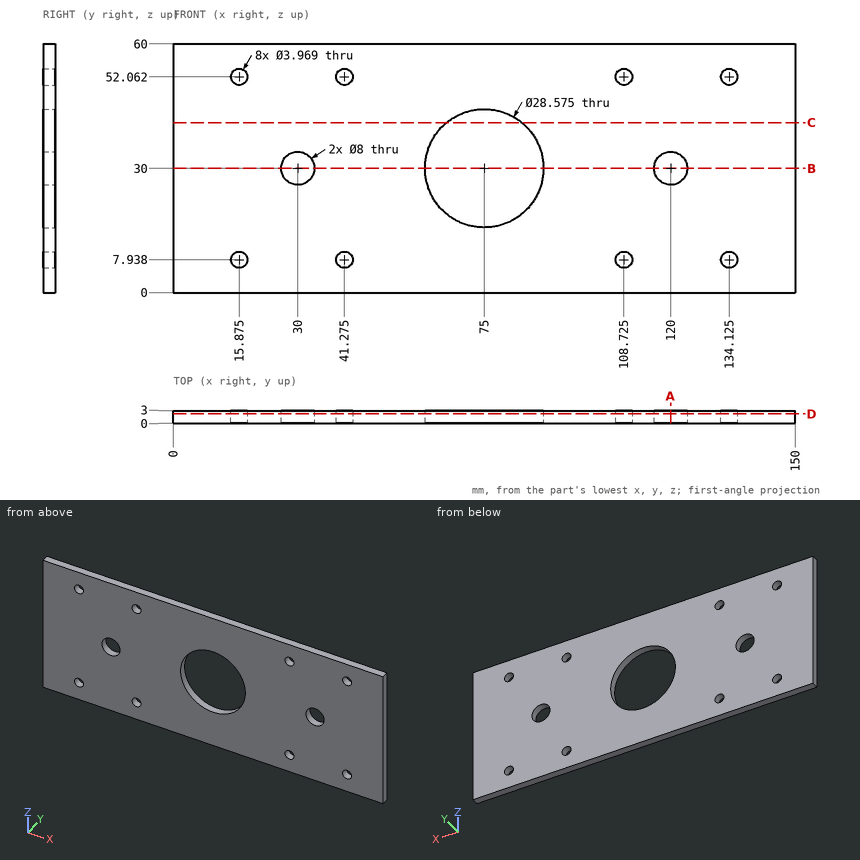
Print and shaded views of the part. All mm, measured from the part's lowest x, y and z. Round coordinates to 2 decimals unless told otherwise and drop trailing zeros. Order: outer loops, then holes, each group sorted by start corner. A loop starts at its lowest first (then second) coordinate and runs counter-clockwise, first axis right, second up.
Q1. Slice it at B-B (z = 30). Write the cut outline in (x, y).
Q2. Slice it at A-A (x = 120). Write the cut outline in (y, z), and give its area (3 significant figures).
Q3. Drop a flat-ended pin along its axis: pin 1 (5 mm diameter, centred on x = 134.12, z = 7.94, fed in from -Y). Give the stop position or say it passes through.
Q4. Wall check: L1, parallel to X at y = 1.9, z = 52; L2, parallel to X at y = 1.45, z = 30; L3, parallel to Z at x = 30, y = 0.75. Give the ranges that are in metal, low to high.
Q5. Slice it at D-D (y = 2.2). State how many separate pieces and enclosed holes the cut face has, and give its area (3 significant figures).
Q6. Slice it at C-C (z = 41). Write the cut outline in (x, y).
Results below:
1. outline: (0, 0) - (26, 0) - (26, 3) - (0, 3) - close; (34, 0) - (60.71, 0) - (60.71, 3) - (34, 3) - close; (89.29, 0) - (116, 0) - (116, 3) - (89.29, 3) - close; (124, 0) - (150, 0) - (150, 3) - (124, 3) - close
2. outline: (0, 0) - (3, 0) - (3, 26) - (0, 26) - close; (0, 34) - (3, 34) - (3, 60) - (0, 60) - close
2. area: 156 mm2
3. pin 1: stops at y = 0
4. L1: x = 0 to 13.89, 17.86 to 39.29, 43.26 to 106.74, 110.71 to 132.14, 136.11 to 150
4. L2: x = 0 to 26, 34 to 60.71, 89.29 to 116, 124 to 150
4. L3: z = 0 to 26, 34 to 60
5. separate pieces: 1
5. enclosed holes: 11
5. area: 8,160 mm2
6. outline: (0, 0) - (65.88, 0) - (65.88, 3) - (0, 3) - close; (84.12, 0) - (150, 0) - (150, 3) - (84.12, 3) - close
